```python
from build123d import *

# Parameters (mm, degrees)
SKETCH1_R           = 5.25
SKETCH1_R_2         = 2.5
BOSS_EXTRUDE1_DEPTH = 1.6
SKETCH3_W           = 120
SKETCH3_H           = 1.6
BOSS_EXTRUDE3_DEPTH = 60
SKETCH4_R           = 3
SKETCH4_R_2         = 1.55
SKETCH4_R_3         = 1.75
CUT_EXTRUDE1_DEPTH  = 10
SKETCH6_R           = 1.7
CUT_EXTRUDE2_DEPTH  = 25
SKETCH7_W           = 25.5
SKETCH7_H           = 1.6
BOSS_EXTRUDE4_DEPTH = 25


with BuildPart() as part:
    # Sketch1 → Boss-Extrude1 (new body)
    with BuildSketch(Plane(origin=(0, 0, 0), x_dir=(1, 0, 0), z_dir=(0, 1, 0))):
        Polygon((34.5, -12), (34.5, 13.5), (11, 13.5), (11, -12), (-60, -12), (-60, 20), (60, 20), (60, -12), align=None)
        with Locations(Location((0, 0, 0), (0, 0, 270))):
            Circle(SKETCH1_R, mode=Mode.SUBTRACT)
        with Locations(Location((-43, 0, 0), (0, 0, 270))):
            Circle(SKETCH1_R_2, mode=Mode.SUBTRACT)
        with Locations(Location((43, 0, 0), (0, 0, 90))):
            Circle(SKETCH1_R_2, mode=Mode.SUBTRACT)
    boss_extrude1 = extrude(amount=BOSS_EXTRUDE1_DEPTH)

    # Sketch3 → Boss-Extrude3 (add)
    with BuildSketch(Plane.XZ):
        with Locations((0, 12.8)):
            Rectangle(SKETCH3_W, SKETCH3_H)
    extrude(amount=-BOSS_EXTRUDE3_DEPTH)

    # Mirror1: Boss-Extrude1 across plane
    add(boss_extrude1.mirror(Plane.ZX.offset(30)))

    # Sketch4 → Cut-Extrude1 (cut)
    with BuildSketch(Plane.XY.offset(12)):
        with Locations(Location((22.75, 26.5, 0), (0, 0, 180))):
            Circle(SKETCH4_R)
        with Locations(Location((31.5, 6.5, 0), (0, 0, 180))):
            Circle(SKETCH4_R_2)
        with Locations(Location((14, 6.5, 0), (0, 0, 180))):
            Circle(SKETCH4_R_2)
        with Locations(Location((22.75, 15, 0), (0, 0, 180))):
            Circle(SKETCH4_R_3)
    extrude(amount=CUT_EXTRUDE1_DEPTH, mode=Mode.SUBTRACT)

    # Sketch6 → Cut-Extrude2 (cut)
    with BuildSketch(Plane(origin=(124.244525073, 40.7, 12), x_dir=(1, 0, 0), z_dir=(0, 0, 1))):
        with Locations(Location((-175.244525073, 9.7, 0), (0, 0, 180))):
            Circle(SKETCH6_R)
        with Locations(Location((-146.994525073, 9.7, 0), (0, 0, 180))):
            Circle(SKETCH6_R)
        with Locations(Location((-101.494525073, 9.7, 0), (0, 0, 180))):
            Circle(SKETCH6_R)
        with Locations(Location((-73.244525073, 9.7, 0), (0, 0, 180))):
            Circle(SKETCH6_R)
        with Locations((-175.244525073, -34.5)):
            Circle(SKETCH6_R)
        with Locations((-146.994525073, -34.5)):
            Circle(SKETCH6_R)
        with Locations(Location((-101.494525073, -34.5, 0), (0, 0, 180))):
            Circle(SKETCH6_R)
        with Locations(Location((-73.244525073, -34.5, 0), (0, 0, 180))):
            Circle(SKETCH6_R)
    extrude(amount=CUT_EXTRUDE2_DEPTH, mode=Mode.SUBTRACT)

    # Sketch7 → Boss-Extrude4 (add)
    with BuildSketch(Plane.ZY.offset(-34.5)):
        with Locations((-0.75, 59.2)):
            Rectangle(SKETCH7_W, SKETCH7_H)
    extrude(amount=BOSS_EXTRUDE4_DEPTH)


solid = part.part
```
Source: CAD feature listing. Evaluate the final solid. Frame: model axes, mm. A direction names the side the tool comes from. Round coordinates to 2 decimals unless told otherwise and drop trailing zeros. Write each loop counter-clockwise with the first axis right and the second up, starting at its lowest first coordinate (ties: lowest second). Pieces come first, ordered by that corner, then holes. Notation, with made-up numbers: M 83,74 L 120,74 A16 ccw 120,97 Z; hole C -6.5,67 d5. An arc over 180 degrees is marked long. Answer as a JSON object with one key per item and string values. Group by question number.
(1) Mould query, pull axis Y, two halves, no side actions, for faces 3 (the cylindrical face through (1.6, 0.8, 5)), 4 (the cylindrical face through (-52.25, 7.35, 12.79)). Classes: +Y half, -Y half, draft (parallel to the pull), parting line (faces both ways), or undercut.
(2) Section query B-B on x = -51. Output: boundary loops of the cut face in (y, z).
(3) Section query C-C on y = 15. Output: boundary loops of the cut face in (x, z), then the cut area to 3 significant figures.
(4) Reachability of faces 1 (the cylindrical face through (-23.53, 51.91, 12.79)), 2 (the flat face through (1, 58.4, -8)) from +Z, -Z, +X, -X, +Y, -Y: full face, straight path, thin tool, end or side. Return the list, or none.
(5) Section query D-D on z = -4. Output: boundary loops of the cut face in (x, y), then the cut area to 3 significant figures.
(6) Ray query, line 1 (Y direction, x = -51, z = 12.7); line 2 (X direction, y = 59, z = 0); line 3 (Y direction, x = 6.5, z = 7.5). Return the intervals inside material, ascending. Write a range as [from, to].
(7) Section query A-A on y = 50.4. Output: boundary loops of the cut face in (x, z).
(8) First-contact query: pin 1 (3 mm diameter, centred on x = 22.75, y = 15, fed in from +Z); pin 2 (4.5 mm diameter, centred on x = 51, y = 6.2, fed in from +Z); pin 3 (3.5 mm diameter, centred on x = 31.5, y = 6.5, fed in from -Z). Flat tips, straight axial feed; report the tip coordinate or a pass-through.
Computed values:
{
 "1": {"face 3": "draft", "face 4": "undercut"},
 "2": {"outline": "M 0,-20 L 1.6,-20 L 1.6,12 L 4.5,12 L 4.5,13.6 L 0,13.6 Z; M 7.9,12 L 48.7,12 L 48.7,13.6 L 7.9,13.6 Z; M 52.1,12 L 58.4,12 L 58.4,-20 L 60,-20 L 60,13.6 L 52.1,13.6 Z"},
 "3": {"outline": "M -60,12 L 21,12 L 21,13.6 L -60,13.6 Z; M 24.5,12 L 60,12 L 60,13.6 L 24.5,13.6 Z", "area": "186 mm^2"},
 "4": {"face 1": "+Z, -Z", "face 2": "-Z, +X, -X"},
 "5": {"outline": "M -60,0 L -3.4,0 L -3.4,1.6 L -60,1.6 Z; M -60,58.4 L -3.4,58.4 L -3.4,60 L -60,60 Z; M 3.4,0 L 11,0 L 11,1.6 L 3.4,1.6 Z; M 3.4,58.4 L 60,58.4 L 60,60 L 3.4,60 Z; M 34.5,0 L 60,0 L 60,1.6 L 34.5,1.6 Z", "area": "325 mm^2"},
 "6": {"line 1": "[0, 4.5], [7.9, 48.7], [52.1, 60]", "line 2": "[-60, -45.5], [-40.5, -5.25], [5.25, 40.5], [45.5, 60]", "line 3": "[0, 1.6], [58.4, 60]"},
 "7": {"outline": "M -60,12 L -52.7,12 L -52.7,13.6 L -60,13.6 Z; M -49.3,12 L -24.45,12 L -24.45,13.6 L -49.3,13.6 Z; M -21.05,12 L 21.05,12 L 21.05,13.6 L -21.05,13.6 Z; M 24.45,12 L 49.3,12 L 49.3,13.6 L 24.45,13.6 Z; M 52.7,12 L 60,12 L 60,13.6 L 52.7,13.6 Z"},
 "8": {"pin 1": "through", "pin 2": "z = 13.6", "pin 3": "z = 12"}
}
